Work out the finished part from the listing and answer in its coordinate system (mm). Face numbers are marked on the shaded views. A direction names the side the tool comes from. Give positions to 0.01 mm unless a question says otherwise; leave off trailing zeros. Order: outer loops, then holes, each group sorted by start corner. A loop starts at its lowest first (then second) coordinate and runs counter-clockwise, first axis right, second up.
```python
from build123d import *

# Parameters (mm, degrees)
F1_DEPTH      = 508
F1_DEPTH_BACK = 158.75
F3_D          = 26.9875
F3_DEPTH      = 25.4
F3_TIP        = 8.107862978
F5_D          = 26.9875
F5_DEPTH      = 25.4
F5_TIP        = 8.107862978


# Not quite as in the source:
# - a feature names something its author has since deleted; it is built from what else it names


with BuildPart() as f1:
    # F0 (on Front) → F1 (new body, two sides)
    with BuildSketch(Plane.XZ) as f1_sk:
        with BuildLine():
            Line((127, -228.6), (127, -203.2))
            Line((127, -203.2), (12.065, -203.2))
            ThreePointArc((12.065, -203.2), (10.2689487758, -202.4560512242), (9.525, -200.66))
            Line((9.525, -200.66), (9.525, 200.66))
            ThreePointArc((9.525, 200.66), (10.2689487758, 202.4560512242), (12.065, 203.2))
            Line((12.065, 203.2), (127, 203.2))
            Line((127, 203.2), (127, 228.6))
            Line((127, 228.6), (-127, 228.6))
            Line((-127, 228.6), (-127, 203.2))
            Line((-127, 203.2), (-12.065, 203.2))
            ThreePointArc((-12.065, 203.2), (-10.2689487758, 202.4560512242), (-9.525, 200.66))
            Line((-9.525, 200.66), (-9.525, -200.66))
            ThreePointArc((-9.525, -200.66), (-10.2689487758, -202.4560512242), (-12.065, -203.2))
            Line((-12.065, -203.2), (-127, -203.2))
            Line((-127, -203.2), (-127, -228.6))
            Line((-127, -228.6), (127, -228.6))
        make_face()
    extrude(amount=F1_DEPTH)
    extrude(f1_sk.sketch, amount=-F1_DEPTH_BACK)

    # F3
    with Locations(Plane.XY.offset(228.6)):
        with Locations((63.5, 127), (63.5, 63.5), (63.5, 0), (-63.5, 0), (-63.5, 63.5), (-63.5, 127)):
            Hole(F3_D / 2, depth=F3_DEPTH)
            with Locations((0, 0, -(F3_DEPTH + F3_TIP / 2))):  # 118° drill point
                Cone(0, F3_D / 2, F3_TIP, mode=Mode.SUBTRACT)

    # F5
    with Locations(Plane(origin=(0, 0, -228.6), x_dir=(1, 0, 0), z_dir=(0, 0, -1))):
        with Locations((63.5, -127), (63.5, -63.5), (63.5, 0), (-63.5, 0), (-63.5, -63.5), (-63.5, -127)):
            Hole(F5_D / 2, depth=F5_DEPTH)
            with Locations((0, 0, -(F5_DEPTH + F5_TIP / 2))):  # 118° drill point
                Cone(0, F5_D / 2, F5_TIP, mode=Mode.SUBTRACT)


solid = f1.part
```
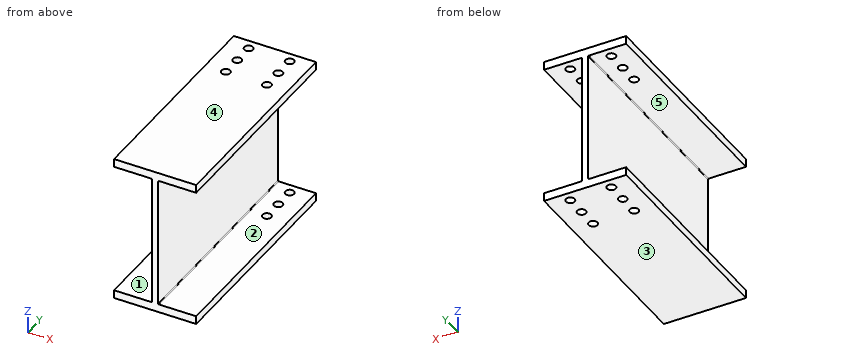
1. Given P1, Ø2, axis at y = -236, z = -172.5, coming from the +X side (3 decimals); P2, Ø24.5, axis at x = 63.5, y = 127, coming from the +Z side; P3, Ø8, axis at y = -418, z = 117.5, coming from the -X side (3 decimals), each flat-ended and moving along its own axis, determine where each tip first touches the part or whether it passes through.
Findings below:
P1: stops at x = 9.525
P2: passes through
P3: stops at x = -9.525
2. The part is cut by section D-D (y = -243.5). Write down the section's boundary in (x, z) (3 decimals), then the cut area to 3 significant figures.
Findings below:
outline: (-127, -228.6) - (127, -228.6) - (127, -203.2) - (12.065, -203.2) arc R2.54 cw to (9.525, -200.66) - (9.525, 200.66) arc R2.54 cw to (12.065, 203.2) - (127, 203.2) - (127, 228.6) - (-127, 228.6) - (-127, 203.2) - (-12.065, 203.2) arc R2.54 cw to (-9.525, 200.66) - (-9.525, -200.66) arc R2.54 cw to (-12.065, -203.2) - (-127, -203.2) - close
area: 20,700 mm2
3. The part is cut by section A-A (x = 63.5). State how many separate pieces and enclosed holes the cut face has, then the cut area to 3 significant figures.
Findings below:
separate pieces: 8
enclosed holes: 0
area: 29,800 mm2
4. The part is cut by section B-B (x = -32.5). Write down the section's boundary in (y, z).
Findings below:
outline: (-508, -228.6) - (158.75, -228.6) - (158.75, -203.2) - (-508, -203.2) - close; (-508, 203.2) - (158.75, 203.2) - (158.75, 228.6) - (-508, 228.6) - close
5. Straight lines are drawn through the part: probe 1 along Y at (x, z) = (-63.5, 211.5); probe 2 along X at (y, z) = (0, 215.25); probe 3 along Z at (x, y) = (37.5, -66). For each, find the intervals that lie inside material, in ascending order.
Findings below:
probe 1: y = -508 to -13.49, 13.49 to 50.01, 76.99 to 113.51, 140.49 to 158.75
probe 2: x = -127 to -76.99, -50.01 to 50.01, 76.99 to 127
probe 3: z = -228.6 to -203.2, 203.2 to 228.6
6. Which of the six approach directions +Z, -Z, +X, -X, +Y, -Y give full straight-line access (tool end or side, diameter ignored) to the marked faces 1 and 2?
Findings below:
face 1: -X, +Y, -Y
face 2: +X, +Y, -Y
7. The mould has two halves that part along Z. Classify the marked faces 3, 4 and 5: pulls with the +Z half, pulls with the -Z half, needs draft (parallel to the pull), parting line crosses it, or undercut.
Findings below:
face 3: pulls with the -Z half
face 4: pulls with the +Z half
face 5: undercut
